Read the model definition and answer for the solid it produces. Units are mm, in the model's axes. A direction names the side the tool comes from. Give positions to 0.01 mm unless a question says otherwise; leave off trailing zeros. Write each loop counter-clockwise with the first axis right and the second up, starting at its lowest first coordinate (ties: lowest second). Pieces come first, ordered by that corner, then holes. Notation, with made-up numbers: M 48,70.25 L 69,70.25 A24 cw 69,83.25 Z; hole C 78.25,75.5 d9. An arc over 180 degrees is marked long. Answer as CSV lines item,"result". Start each with the question number.
```python
from build123d import *

# Parameters (mm, degrees)
SKETCH_1_R          = 35
EXTRUDE_1_DEPTH     = 30
SKETCH_2_W          = 98.5
SKETCH_2_H          = 70
EXTRUDE_2_DEPTH     = 3
FILLET_1_R          = 10
FILLET_2_R          = 30
FILLET_3_R          = 30
SKETCH_3_R          = 1.3
SKETCH_3_R_2        = 1.252848492
CUT_EXTRUDE_1_DEPTH = 3
SKETCH_4_R          = 14
EXTRUDE_3_DEPTH     = 22


with BuildPart() as part:
    # 스케치1 → 보스-돌출1 (new body)
    with BuildSketch(Plane(origin=(0, 0, 0), x_dir=(1, 0, 0), z_dir=(0, 1, 0))):
        Circle(SKETCH_1_R)
    extrude(amount=EXTRUDE_1_DEPTH)

    # 스케치2 → 보스-돌출2 (add)
    with BuildSketch(Plane.XZ):
        with Locations((14.25, 0)):
            Rectangle(SKETCH_2_W, SKETCH_2_H)
    extrude(amount=EXTRUDE_2_DEPTH)

    # 필렛1
    fillet_1_edges = [part.edges().sort_by_distance(p)[0] for p in [
        (-35, -1.5, 35),
        (-35, -1.5, -35),
    ]]
    fillet(fillet_1_edges, radius=FILLET_1_R)

    # 필렛2
    fillet_2_edges = [part.edges().sort_by_distance(p)[0] for p in [
        (63.5, -1.5, -35),
    ]]
    fillet(fillet_2_edges, radius=FILLET_2_R)

    # 필렛3
    fillet_3_edges = [part.edges().sort_by_distance(p)[0] for p in [
        (63.5, -1.5, 35),
    ]]
    fillet(fillet_3_edges, radius=FILLET_3_R)

    # 스케치3 → 컷-돌출1 (cut)
    with BuildSketch(Plane(origin=(0, 0, 0), x_dir=(1, 0, 0), z_dir=(0, 1, 0))):
        with Locations((-28, 28)):
            Circle(SKETCH_3_R)
        with Locations((-28, -28.00420951)):
            Circle(SKETCH_3_R_2)
        with Locations((42, 20)):
            Circle(SKETCH_3_R)
        with Locations((42, -20)):
            Circle(SKETCH_3_R)
    extrude(amount=-CUT_EXTRUDE_1_DEPTH, mode=Mode.SUBTRACT)

    # 스케치4 → 보스-돌출3 (add)
    with BuildSketch(Plane.XZ.offset(3)):
        with Locations((45, 0)):
            Circle(SKETCH_4_R)
    extrude(amount=EXTRUDE_3_DEPTH)


solid = part.part
```
1. Determine the mould class of faces 1 (the face through (54.479, -1.521, -26.445)), 2 (the face through (45, 0, 0)), 3 (the face through (40.7, -1.48, 19.94)) for opening direction X: +X half, -X half, draft (parallel to the pull), parting line (faces both ways), or undercut.
2. Find section B-B on z = -20. Determine the outline of the cut face in (x, y).
3. For faces 4 (the face through (0, 30, 0)), 5 (the face through (-27, 0, -26)), 6 (the face through (-27, 0, 27)), 7 (the face through (-28, 15, 21)), 8 (the face through (31.014, -13.846, 0.616)), determine the directions among +Z, -Z, +X, -X, +Y, -Y from which every point of the face is accessible in a straight line to the end or side of a thin tool.
4. Find section A-A on x = 42. Determine the outline of the cut face in (y, z), then the cut area to 3 significant figures.
5. Find section D-D on z = 2. Determine the outline of the cut face in (x, y).
6. Find the intervals of material crossed by line 1 (Y direction, x = -18, z = -14); line 2 (X direction, y = 24.5, z = 0); line 3 (Y direction, x = 38, z = -17), in increasing order. Write a range as [from, to].
7. Given pin 1 (8 mm diameter, centred on x = 35.5, y = -15, fed in from +Z); pin 2 (8 mm diameter, centred on x = -2.5, z = 9.5, fed in from -Y); pin 3 (4 mm diameter, centred on x = 42, z = 20, fed in from +Y), each flat-ended and moving along its own axis, determine where each tip first touches the part or whether it passes through.
8. Find section C-C on x = -5. Determine the outline of the cut face in (y, z).
Computed:
1,face 1,"+X half"
1,face 2,"draft"
1,face 3,"undercut"
2,outline,"M -35,-3 L 40.7,-3 L 40.7,0 L 28.72,0 L 28.72,30 L -28.72,30 L -28.72,0 L -35,0 Z; M 43.3,-3 L 59.48,-3 L 59.48,0 L 43.3,0 Z"
3,face 4,"+Z, -Z, +X, -X, +Y"
3,face 5,"-Z, -X, +Y"
3,face 6,"+Z, -X, +Y"
3,face 7,"+Y"
3,face 8,"-Y"
4,outline,"M -25,-13.67 L -3,-13.67 L -3,-18.7 L 0,-18.7 L 0,18.7 L -3,18.7 L -3,13.67 L -25,13.67 Z; M -3,-33.77 L 0,-33.77 L 0,-21.3 L -3,-21.3 Z; M -3,21.3 L 0,21.3 L 0,33.77 L -3,33.77 Z"
4,area,"789 mm^2"
5,outline,"M -35,-3 L 31.14,-3 L 31.14,-25 L 58.86,-25 L 58.86,-3 L 63.5,-3 L 63.5,0 L 34.94,0 L 34.94,30 L -34.94,30 L -34.94,0 L -35,0 Z"
6,line 1,"y = [-3, 30]"
6,line 2,"x = [-35, 35]"
6,line 3,"y = [-3, 0]"
7,pin 1,"stops at z = 12.87"
7,pin 2,"stops at y = -3"
7,pin 3,"stops at y = 0"
8,outline,"M -3,-35 L 0,-35 L 0,-34.64 L 30,-34.64 L 30,34.64 L 0,34.64 L 0,35 L -3,35 Z"
